Could you check a few things on this model? Use its own coordinates, in mm. A direction names the side the tool comes from. Coordinates: 2 decimals unless noted, no trailing zeros. Order: outer loops, then holes, each group sorted by start corner. A loop starts at its lowest first (then second) coordinate and runs counter-clockwise, first axis right, second up.
Autodesk Inventor part; units mm, degrees
ref_plane "YZ Plane" through (0, 0, 0) normal (1, 0, 0) x (0, 1, 0)
ref_plane "XZ Plane" through (0, 0, 0) normal (0, 1, 0) x (-1, 0, 0)
ref_plane "XY Plane" through (0, 0, 0) normal (0, 0, 1) x (1, 0, 0)
sketch "Sketch1" plane through (0, 0, 0) normal (0, 0, 1) x (1, 0, 0)
  circle A0 centre (0, 0) radius 8
  circle A1 centre (0, 0) radius 13
  line L0 (0, 13) -> (35, 13)
  line L1 (35, 13) -> (35, -13)
  line L2 (35, -13) -> (0, -13)
  dimension "d0" = 16
  dimension "d1" = 26
  dimension "d2" = 48
extrude "Extrusion1" add sketch "Sketch1" against normal blind 50
sketch "Sketch2" plane through (0, 0, 0) normal (0, 0, 1) x (1, 0, 0)
  circle A0 centre (0, 0) radius 8
  line L0 (35, 13) -> (0, 13)
  line L1 (10, 10.5) -> (28, 10.5)
  line L2 (28, 10.5) -> (28, -10.5)
  line L3 (28, -10.5) -> (10, -10.5)
  line L4 (10, -10.5) -> (10, 10.5)
  dimension "d5" = 18
  dimension "d6" = 21
  dimension "d7" = 10
  dimension "d8" = 2.5
extrude "Extrusion2" cut sketch "Sketch2" against normal up to surface (50 mm away) contours L1 L2 L3 L4
sketch "Sketch3" plane through (0, 13, 0) normal (0, 1, 0) x (1, 0, 0)
  line L0 (0, 50) -> (35, 50)
  line L1 (0, 0) -> (0, 50)
  circle A0 centre (25, 32.5) radius 2
  circle A1 centre (25, 17.5) radius 2
  line L2 (-8, 50) -> (8, 50)
  line L3 (8, 0) -> (-8, 0)
  dimension "d11" = 4
  dimension "d12" = 4
  dimension "d13" = 15
  dimension "d14" = 25
  dimension "d15" = 17.5
extrude "Extrusion3" cut sketch "Sketch3" along normal blind 50 and the other way blind 29.25
sketch "Sketch4" plane through (35, -13, 0) normal (1, 0, 0) x (0, 0, -1)
  line L0 (0, 0) -> (0, 26)
  line L1 (0, 0) -> (50, 0)
  line L2 (18, 2.5) -> (32, 2.5)
  line L3 (32, 2.5) -> (32, 23.5)
  line L4 (32, 23.5) -> (18, 23.5)
  line L5 (18, 23.5) -> (18, 2.5)
  point P0 (0, 13)
  dimension "d20" = 14
  dimension "d21" = 21
  dimension "d22" = 18
  dimension "d23" = 2.5
extrude "Extrusion4" cut sketch "Sketch4" against normal up to surface (7 mm away)
chamfer "Chamfer1" distance 5 angle 45 2 edges at (28, 0, -32) (28, 0, -18)
sketch "Sketch5" plane through (35, -13, 0) normal (1, 0, 0) x (0, 0, -1)
  line L0 (0, 0) -> (50, 0)
  line L1 (50, 26) -> (50, 0)
  line L2 (0, 26) -> (50, 26)
  circle A0 centre (25, 33) radius 4
  circle A1 centre (25, -7) radius 4
  line L3 (0, 26) -> (50, 26)
  line L4 (17, 26) -> (17, 40)
  line L5 (17, 40) -> (33, 40)
  line L6 (33, 40) -> (33, 26)
  line L7 (0, 0) -> (50, 0)
  line L8 (17, 0) -> (17, -14)
  line L9 (17, -14) -> (33, -14)
  line L10 (33, -14) -> (33, 0)
  point P0 (0, 13)
  dimension "d29" = 8
  dimension "d30" = 8
  dimension "d31" = 25
  dimension "d32" = 40
  dimension "d33" = 7
  dimension "d34" = 14
  dimension "d35" = 14
  dimension "d36" = 8
  dimension "d37" = 8
extrude "Extrusion5" add sketch "Sketch5" against normal blind 22
properties part number "XEndTop"
Item 1: Suppose I cut it at C-C (y = 20). List the corners of the cut face in (x, z) for me.
Item 2: Which directions (+Z, -Z, +X, -X, +Y, -Y) give clear straight access to the entire face, cutting with the end or side of a thin tool? Please do faces 5 (the face through (13, 22, -21)), 6 (the face through (13, -18, -21)), 7 (the face through (28, 0, -43)), 8 (the face through (24.566, -11.733, -30.548)), 9 (the face through (24, 20, -33)).
Item 3: I need wall thicknesses on line 1 (Z direction, x = 25, y = 11.8); line 2 (Y direction, x = 18.5, z = -25); line 3 (Y direction, x = 13, z = -40.5). Which ranges of each line are inside material? Lowest first, please.
Item 4: Thinking about a two-plate mould opening in Y: for faces 1 (the face through (20, -10.5, -25)), 2 (the face through (31, 0, -34)), 3 (the face through (5, 9, 0)), 4 (the face through (24, 27, -25)), which applies, +Y half, -Y half, draft (parallel to the pull), parting line (faces both ways), or undercut?
Item 5: For pin 1 Ø5 at (y, z) = (-16, -43) entering from +X; pin 2 Ø5 at (y, z) = (-19.5, -29) entering from -X; pin 3 Ø15.5 at (x, y) = (21.5, 23) entering from -Z; pin 4 Ø1 at (x, z) = (20, -13.5) entering from +Y, each with a flat end and sliding along its axis, tell me the tip position at first contact or that it passes through.
Item 6: Suppose I cut it at A-A (z = -25). List the corners of the cut face in (x, y) for me, and give its area (3 significant figures).
Item 7: Suppose I cut it at D-D (x = 11). List the corners of the cut face in (y, z) for me, and give its area (3 significant figures).
Item 8: Suppose I cut it at B-B (x = 25). Count the separate pieces of the cut face and the enclosed holes in it, and give its area (3 significant figures).
Geometry results:
1. outline: (13, -33) - (35, -33) - (35, -29) - (13, -29) - close; (13, -21) - (35, -21) - (35, -17) - (13, -17) - close
2. face 5: +Z, -Z, -X, +Y
2. face 6: +Z, -Z, -X, -Y
2. face 7: +Z, -Z
2. face 8: none
2. face 9: -Z, +X, -X, +Y
3. line 1: z = -50 to -34.5, -30.5 to -19.5, -15.5 to 0
3. line 2: y = -27 to -24, -16 to -10.5, 10.5 to 16, 24 to 27
3. line 3: y = -13 to -10.5, 10.5 to 13
4. face 1: undercut
4. face 2: undercut
4. face 3: draft
4. face 4: +Y half
5. pin 1: passes through
5. pin 2: stops at x = 13
5. pin 3: stops at z = -33
5. pin 4: stops at y = 13
6. outline: (0, -13) - (13, -13) - (13, -16) - (35, -16) - (35, -10.5) - (10, -10.5) - (10, 10.5) - (35, 10.5) - (35, 16) - (13, 16) - (13, 13) - (0, 13) arc R13 ccw to start; (13, -27) - (35, -27) - (35, -24) - (13, -24) - close; (13, 24) - (35, 24) - (35, 27) - (13, 27) - close; hole circle Ø16 at (0, 0)
6. area: 713 mm2
7. outline: (-13, -50) - (-10.5, -50) - (-10.5, 0) - (-13, 0) - close; (10.5, -50) - (13, -50) - (13, 0) - (10.5, 0) - close
7. area: 250 mm2
8. separate pieces: 6
8. enclosed holes: 2
8. area: 557 mm2
